from build123d import *

# Parameters (mm, degrees)
SKETCH_1_R          = 1.5
SKETCH_1_R_2        = 10
SKETCH_1_R_3        = 4.5
SKETCH_1_R_4        = 2
SKETCH_1_W          = 8.05
SKETCH_1_H          = 4.05
SKETCH_1_W_2        = 4.05
SKETCH_1_H_2        = 8.05
EXTRUDE_1_DEPTH     = 4
SKETCH_2_W          = 132
SKETCH_2_H          = 24
CUT_EXTRUDE_1_DEPTH = 4
CUT_EXTRUDE_2_DEPTH = 4


with BuildPart() as part:
    # 草图1 → 凸台-拉伸1 (new body)
    with BuildSketch(Plane.XY):
        Polygon((47.027428163, 101.054738201), (113.027428163, 101.054738201), (113.027428163, -30.945261799), (-18.972571837, -30.945261799), (-18.972571837, 101.054738201), align=None)
        with Locations((47.027428163, 96.155233813)):
            Circle(SKETCH_1_R, mode=Mode.SUBTRACT)
        with Locations((108.127923775, 35.054738201)):
            Circle(SKETCH_1_R, mode=Mode.SUBTRACT)
        with Locations((47.027428163, 35.054738201)):
            Circle(SKETCH_1_R_2, mode=Mode.SUBTRACT)
        with Locations((47.027428163, 15.054738201)):
            Circle(SKETCH_1_R_3, mode=Mode.SUBTRACT)
        with Locations((27.027428163, 15.054738201)):
            Circle(SKETCH_1_R_4, mode=Mode.SUBTRACT)
        with Locations((27.027428163, 55.054738201)):
            Circle(SKETCH_1_R_4, mode=Mode.SUBTRACT)
        with Locations((67.027428163, 55.054738201)):
            Circle(SKETCH_1_R_4, mode=Mode.SUBTRACT)
        with Locations((67.027428163, 15.054738201)):
            Circle(SKETCH_1_R_4, mode=Mode.SUBTRACT)
        with Locations((47.027428163, -26.045757411)):
            Circle(SKETCH_1_R, mode=Mode.SUBTRACT)
        with Locations((-14.073067448, 35.054738201)):
            Circle(SKETCH_1_R, mode=Mode.SUBTRACT)
        with Locations((14.027428163, 96.155233813)):
            Rectangle(SKETCH_1_W, SKETCH_1_H, mode=Mode.SUBTRACT)
        with Locations((80.027428163, 96.155233813)):
            Rectangle(SKETCH_1_W, SKETCH_1_H, mode=Mode.SUBTRACT)
        with Locations((108.127923775, 68.054738201)):
            Rectangle(SKETCH_1_W_2, SKETCH_1_H_2, mode=Mode.SUBTRACT)
        with Locations((108.127923775, 2.054738201)):
            Rectangle(SKETCH_1_W_2, SKETCH_1_H_2, mode=Mode.SUBTRACT)
        with Locations((80.027428163, -26.045757411)):
            Rectangle(SKETCH_1_W, SKETCH_1_H, mode=Mode.SUBTRACT)
        with Locations((14.027428163, -26.045757411)):
            Rectangle(SKETCH_1_W, SKETCH_1_H, mode=Mode.SUBTRACT)
        with Locations((-14.073067448, 2.054738201)):
            Rectangle(SKETCH_1_W_2, SKETCH_1_H_2, mode=Mode.SUBTRACT)
        with Locations((-14.073067448, 68.054738201)):
            Rectangle(SKETCH_1_W_2, SKETCH_1_H_2, mode=Mode.SUBTRACT)
    extrude(amount=EXTRUDE_1_DEPTH)

    # 草图2 → 切除-拉伸1 (cut)
    with BuildSketch(Plane(origin=(0, 0, 0), x_dir=(-1, 0, 0), z_dir=(0, 0, -1))):
        with Locations((-47.027428163, -18.945261799)):
            Rectangle(SKETCH_2_W, SKETCH_2_H)
    extrude(amount=-CUT_EXTRUDE_1_DEPTH, mode=Mode.SUBTRACT)

    # 草图3 → 切除-拉伸2 (cut)
    with BuildSketch(Plane(origin=(0, 0, 0), x_dir=(-1, 0, 0), z_dir=(0, 0, -1))):
        with BuildLine():
            Line((-72.542129808, 30.054738201), (-99.515674348, 30.054738201))
            ThreePointArc((-99.515674348, 30.054738201), (-100.941091534, 29.457658671), (-101.515421297, 28.022924045))
            Line((-101.515421297, 28.022924045), (-101.255391029, 11.678164385))
            ThreePointArc((-101.255391029, 11.678164385), (-100.412595688, 10.078579455), (-98.624288606, 9.812245613))
            Line((-98.624288606, 9.812245613), (-81.193952996, 15.611132086))
            ThreePointArc((-81.193952996, 15.611132086), (-80.304662874, 16.20977419), (-79.852257763, 17.181648105))
            ThreePointArc((-79.852257763, 17.181648105), (-77.616411007, 22.596186492), (-73.230421996, 26.4793987))
            ThreePointArc((-73.230421996, 26.4793987), (-72.353458134, 27.433018894), (-72.244921555, 28.724017307))
            ThreePointArc((-72.244921555, 28.724017307), (-72.402250484, 29.387429123), (-72.542129808, 30.054738201))
        make_face()
        with BuildLine():
            Line((-12.86090333, 15.611132086), (4.569432279, 9.812245613))
            ThreePointArc((4.569432279, 9.812245613), (6.357739361, 10.078579455), (7.200534703, 11.678164385))
            Line((7.200534703, 11.678164385), (7.46056497, 28.022924045))
            ThreePointArc((7.46056497, 28.022924045), (6.886235208, 29.457658671), (5.460818021, 30.054738201))
            Line((5.460818021, 30.054738201), (-21.512726519, 30.054738201))
            ThreePointArc((-21.512726519, 30.054738201), (-21.652605842, 29.387429123), (-21.809934772, 28.724017307))
            ThreePointArc((-21.809934772, 28.724017307), (-21.701398193, 27.433018894), (-20.824434331, 26.4793987))
            ThreePointArc((-20.824434331, 26.4793987), (-16.438445319, 22.596186492), (-14.202598564, 17.181648105))
            ThreePointArc((-14.202598564, 17.181648105), (-13.750193453, 16.20977419), (-12.86090333, 15.611132086))
        make_face()
        with BuildLine():
            Line((4.569432279, -6.945261799), (-101.255391029, -6.945261799))
            Line((-101.255391029, -6.945261799), (-47.866918263, 1.915411357))
            ThreePointArc((-47.866918263, 1.915411357), (-47.027723842, 1.98284019), (-46.189112393, 1.908511437))
            Line((-46.189112393, 1.908511437), (4.569432279, -6.945261799))
        make_face()
        with BuildLine():
            Line((-24.400011165, 41.054738201), (4.444782388, 41.054738201))
            ThreePointArc((4.444782388, 41.054738201), (5.870199575, 41.651817731), (6.444529337, 43.086552357))
            Line((6.444529337, 43.086552357), (6.048067448, 68.007013948))
            Line((6.048067448, 68.007013948), (6.048067448, 74.816525314))
            ThreePointArc((6.048067448, 74.816525314), (4.813434313, 76.664284379), (2.633853886, 76.230738876))
            Line((2.633853886, 76.230738876), (-14.660749072, 58.936135918))
            ThreePointArc((-14.660749072, 58.936135918), (-15.154755521, 58.120835026), (-15.21523446, 57.169467477))
            ThreePointArc((-15.21523446, 57.169467477), (-17.669451156, 47.54286318), (-26.537436176, 43.064746214))
            ThreePointArc((-26.537436176, 43.064746214), (-26.408756591, 42.727441936), (-26.285629249, 42.388071534))
            ThreePointArc((-26.285629249, 42.388071534), (-25.554711704, 41.421745039), (-24.400011165, 41.054738201))
        make_face()
        with BuildLine():
            Line((-100.102923775, 68.007013948), (-100.102923775, 74.816525314))
            ThreePointArc((-100.102923775, 74.816525314), (-98.86829064, 76.664284379), (-96.688710213, 76.230738876))
            Line((-96.688710213, 76.230738876), (-79.394107255, 58.936135918))
            ThreePointArc((-79.394107255, 58.936135918), (-78.900100806, 58.120835026), (-78.839621867, 57.169467477))
            ThreePointArc((-78.839621867, 57.169467477), (-76.385405171, 47.54286318), (-67.517420151, 43.064746214))
            ThreePointArc((-67.517420151, 43.064746214), (-67.646099736, 42.727441936), (-67.769227078, 42.388071534))
            ThreePointArc((-67.769227078, 42.388071534), (-68.500144623, 41.421745039), (-69.654845161, 41.054738201))
            Line((-69.654845161, 41.054738201), (-98.499638715, 41.054738201))
            ThreePointArc((-98.499638715, 41.054738201), (-99.925055902, 41.651817731), (-100.499385664, 43.086552357))
            Line((-100.499385664, 43.086552357), (-100.102923775, 68.007013948))
        make_face()
        with BuildLine():
            Line((-13.7697462, 82.829128974), (-30.109761047, 63.753633363))
            ThreePointArc((-30.109761047, 63.753633363), (-30.792684258, 63.237843917), (-31.628683757, 63.054738201))
            Line((-31.628683757, 63.054738201), (-62.390490848, 63.054738201))
            ThreePointArc((-62.390490848, 63.054738201), (-63.231829728, 63.240310222), (-63.917039651, 63.762589312))
            Line((-63.917039651, 63.762589312), (-80.063513586, 82.838084924))
            ThreePointArc((-80.063513586, 82.838084924), (-80.351392761, 84.971572693), (-78.536964783, 86.130233813))
            Line((-78.536964783, 86.130233813), (-15.28866891, 86.130233813))
            ThreePointArc((-15.28866891, 86.130233813), (-13.471774627, 84.966233311), (-13.7697462, 82.829128974))
        make_face()
    extrude(amount=-CUT_EXTRUDE_2_DEPTH, mode=Mode.SUBTRACT)


solid = part.part
Geometry: final body of the model. Coordinates: model frame, mm. A direction names the side the tool comes from. Give positions to 0.01 mm unless a question says otherwise; leave off trailing zeros. Write each loop counter-clockwise with the first axis right and the second up, starting at its lowest first coordinate (ties: lowest second). Pieces come first, ordered by that corner, then holes.
(1) Cut plane B-B, the plane y = 61. Return loops of the section in (x, z).
(2) Cut plane A-A, the plane x = 90. Return loops of the section in (y, z).
(3) Cut plane C-C, the plane z = 2.85. Give the number of separate pieces and of enclosed holes in the cut face, then the cut area to 3 significant figures.
(4) Ray query, line 1 (Y direction, x = 47, z = 0.4); line 2 (Y direction, x = 76.5, z = 3.1); line 3 (X direction, y = 36, z = 1.05). Return the intervals inside material, ascending.
(5) Mould query, pull axis Y, two halves, no side actions, for faces 4 (the flat face through (107, -6.945, 2)), 5 (the flat face through (-12.048, 2, 2)), 6 (the flat face through (48, 48, 4)). Classes: released by +Y, released by -Y, zero draft, split by the parting line, or undercut.
(6) Access query for faces 1 (the flat face through (-14, 72.08, 2)), 2 (the flat face through (113.027, 48, 2)), 3 (the flat face through (74.935, -2.577, 1.972)). Directions: +Z, -Z, +X, -X, +Y, -Y. A direction counts if a zero-diameter tool reaches every point of the face in a straight line with its end or side. Return the directions, or none.
Values follow:
1. outline: (-18.97, 0) - (-6.16, 0) - (-6.16, 4) - (-18.97, 4) - close; (12.6, 0) - (81.46, 0) - (81.46, 4) - (12.6, 4) - close; (100.21, 0) - (113.03, 0) - (113.03, 4) - (100.21, 4) - close
2. outline: (-5.08, 0) - (12.68, 0) - (12.68, 4) - (-5.08, 4) - close; (30.05, 0) - (41.05, 0) - (41.05, 4) - (30.05, 4) - close; (69.54, 0) - (101.05, 0) - (101.05, 4) - (69.54, 4) - close
3. separate pieces: 1
3. enclosed holes: 20
3. area: 9,800 mm2
4. line 1: y = 1.98 to 10.55, 19.55 to 25.05, 45.05 to 63.05, 86.13 to 94.66, 97.65 to 101.05
4. line 2: y = -2.84 to 23.96, 30.05 to 41.05, 47.69 to 78.63, 86.13 to 94.13, 98.18 to 101.05
4. line 3: x = -18.97 to -15.24, -12.91 to 37.07, 56.98 to 106.96, 109.29 to 113.03
5. face 4: released by -Y
5. face 5: undercut
5. face 6: zero draft
6. face 1: +Z, -Z
6. face 2: +Z, -Z, +X, +Y, -Y
6. face 3: +Z, -Z, -Y
